```python
from build123d import *

# Parameters (mm, degrees)
SKETCH1_R             = 43
BOSS_EXTRUDE1_DEPTH   = 20
SKETCH2_R             = 44
BOSS_EXTRUDE2_DEPTH   = 8
FILLET1_R             = 20
BOSS_EXTRUDE3_DEPTH   = 10
SKETCH5_R             = 2.1
CUT_EXTRUDE1_DEPTH    = 4
CUT_EXTRUDE2_DEPTH    = 5
FILLET2_R             = 3
BOSS_EXTRUDE4_DEPTH   = 10
SKETCH10_R            = 2.1
CUT_EXTRUDE3_DEPTH    = 4
SKETCH11_R            = 3.25
CUT_EXTRUDE4_DEPTH    = 47
CROQUIS1_R            = 2.75
CORTAR_EXTRUIR1_DEPTH = 13
CROQUIS2_R            = 6.4
CORTAR_EXTRUIR2_DEPTH = 10


with BuildPart() as part:
    # Sketch1 → Boss-Extrude1 (new body)
    with BuildSketch(Plane(origin=(0, 0, 0), x_dir=(1, 0, 0), z_dir=(0, 1, 0))):
        with Locations(Location((0, 0, 0), (0, 0, 270))):
            Circle(SKETCH1_R)
    extrude(amount=BOSS_EXTRUDE1_DEPTH)

    # Sketch2 → Boss-Extrude2 (add)
    with BuildSketch(Plane(origin=(0, 20, 0), x_dir=(1, 0, 0), z_dir=(0, 1, 0))):
        with Locations(Location((0, 0, 0), (0, 0, 270))):
            Circle(SKETCH2_R)
    extrude(amount=-BOSS_EXTRUDE2_DEPTH)

    # Fillet1
    # the kernel refuses this fillet: 20 mm, written as the material it adds along each edge
    with BuildSketch(Plane(origin=(0, 12, 0), x_dir=(0, 0, 1), z_dir=(1, 0, 0))) as fillet1_piece_1:
        with BuildLine():
            CenterArc((63, 6.244997998), FILLET1_R, 180, 18.194872339)
            Line((44, 0), (43, 0))
            Line((43, 0), (43, 6.244997998))
        make_face()
    revolve(axis=Axis((0, 12, 0), (0, -1, 0)))

    # Sketch4 → Boss-Extrude3 (add)
    with BuildSketch(Plane.XZ):
        Polygon((28.890073358, 11), (35.011581558, 11), (0, -38.567688166), (-2.046413556, -32.798368085), align=None)
    extrude(amount=BOSS_EXTRUDE3_DEPTH)

    # Sketch5 → Cut-Extrude1 (cut)
    with BuildSketch(Plane(origin=(18.174388611, 0, -12.837275908), x_dir=(-0.576932008090494, 0, -0.8167921755505927), z_dir=(0.8167921755505927, 0, -0.576932008090494))):
        with Locations((-21.184015986, -5)):
            Circle(SKETCH5_R)
        with Locations(Location((23.501785923, -5, 0), (0, 0, 180))):
            Circle(SKETCH5_R)
    extrude(amount=-CUT_EXTRUDE1_DEPTH, mode=Mode.SUBTRACT)

    # Sketch7 → Cut-Extrude2 (cut)
    with BuildSketch(Plane.XZ):
        with BuildLine():
            Line((8.455950561, -5.839980603), (-5.151807084, 3.771706651))
            ThreePointArc((-5.151807084, 3.771706651), (-8.391785298, 4.503949914), (-11.200570041, 2.730713525))
            Line((-11.200570041, 2.730713525), (-20.812257296, -10.87704412))
            ThreePointArc((-20.812257296, -10.87704412), (-21.544500559, -14.117022334), (-19.771264169, -16.925807077))
            Line((-19.771264169, -16.925807077), (-6.163506524, -26.537494332))
            ThreePointArc((-6.163506524, -26.537494332), (-2.92352831, -27.269737595), (-0.114743567, -25.496501205))
            Line((-0.114743567, -25.496501205), (9.496943688, -11.88874356))
            ThreePointArc((9.496943688, -11.88874356), (10.22918695, -8.648765346), (8.455950561, -5.839980603))
        make_face()
    extrude(amount=-CUT_EXTRUDE2_DEPTH, mode=Mode.SUBTRACT)

    # Fillet2
    fillet2_edges = [part.edges().sort_by_distance(p)[0] for p in [
        (0, 20, -44),
    ]]
    fillet(fillet2_edges, radius=FILLET2_R)

    # Sketch8 → Boss-Extrude4 (add)
    with BuildSketch(Plane.XZ):
        Polygon((28.890073358, 11), (-35.011581558, 11), (-31.47988754, 6), (25.35837934, 6), align=None)
    extrude(amount=BOSS_EXTRUDE4_DEPTH)

    # Sketch10 → Cut-Extrude3 (cut)
    with BuildSketch(Plane.XY.offset(11)):
        with Locations((-17.011581558, -5)):
            Circle(SKETCH10_R)
        with Locations((17.011581558, -5)):
            Circle(SKETCH10_R)
    extrude(amount=-CUT_EXTRUDE3_DEPTH, mode=Mode.SUBTRACT)

    # Sketch11 → Cut-Extrude4 (cut)
    with BuildSketch(Plane.XZ):
        with Locations(Location((0, 25, 0), (0, 0, 270))):
            Circle(SKETCH11_R)
    extrude(amount=-CUT_EXTRUDE4_DEPTH, mode=Mode.SUBTRACT)

    # Croquis1 → Cortar-Extruir1 (cut)
    with BuildSketch(Plane(origin=(0, 20, 0), x_dir=(1, 0, 0), z_dir=(0, 1, 0))):
        with Locations(Location((-15, 25, 0), (0, 0, 270))):
            Circle(CROQUIS1_R)
        with Locations(Location((15, 25, 0), (0, 0, 270))):
            Circle(CROQUIS1_R)
        with Locations(Location((15, -25, 0), (0, 0, 270))):
            Circle(CROQUIS1_R)
        with Locations(Location((-15, -25, 0), (0, 0, 270))):
            Circle(CROQUIS1_R)
    extrude(amount=-CORTAR_EXTRUIR1_DEPTH, mode=Mode.SUBTRACT)

    # Croquis2 → Cortar-Extruir2 (cut)
    with BuildSketch(Plane(origin=(0, 20, 0), x_dir=(1, 0, 0), z_dir=(0, 1, 0))):
        with Locations(Location((0, 0, 0), (0, 0, 270))):
            Circle(CROQUIS2_R)
    extrude(amount=-CORTAR_EXTRUIR2_DEPTH, mode=Mode.SUBTRACT)


solid = part.part
```
Can you work these out from the model? Positions are in its coordinate system, mm. A direction names the side the tool comes from. Round coordinates to 2 decimals unless told otherwise and drop trailing zeros. Loops run counter-clockwise (first coordinate to the right, second up) from the corner with the lowest first, then second, coordinate; pieces in that order, holes last. Notation, with made-up numbers: (9, 50) -> (31, 50) arc R31 ccw to (31, 81) -> close; hole circle Ø6 at (48.25, 76). An arc over 180 degrees is marked (long way). One line per item, written item: value. Start each with the question number.
1. If I drill on probe 1 along X at (y, z) = (14.75, 0); probe 2 along Z at (x, y) = (-2.5, 13.25); probe 3 along X at (y, z) = (11.5, -25), over which ranges is the centre line in solid material (lowest first)?
2. If we section it at B-B, the plane z = 0: Write out the boundary of the cut face in (x, y) (3 decimals), then the cut area to 3 significant figures.
3. If we section it at A-A, the plane y = -5: Write out the boundary of the cut face in (x, z).
4. For pin 1 (6.5 mm diameter, centred on x = 17.01, y = -5, fed in from -Z); pin 2 (5 mm diameter, centred on y = -1.5, z = 10, fed in from +X); pin 3 (1.5 mm diameter, centred on x = -32, y = 8.5, fed in from -Z), each with a flat end and sliding along its axis, tell me the tip position at first contact or that it passes through.
5. For faces 5 (the cylindrical face through (-16.04, -6.86, 9.03)), 6 (the flat face through (11.464, -4.93, -13.671)), 7 (the flat face through (-6, 5, -11)), 8 (the flat face through (27.15, -4.97, 6.8)), 9 (the cylindrical face through (15.121, 13.591, 22.253)), which set-ups out of +Z, -Z, +X, -X, +Y, -Y let a thin tool reach every point of the face, with its end or its side?
6. If we mould it in two halves opening along X, with no side actions, what happens to faces 1 (the cylindrical face through (-3.89, 15.07, -5.08)), 2 (the cylindrical face through (-2.971, 2.465, -27.278)), 3 (the flat face through (8, -10, 7)), 4 (the flat face through (-33.27, -4.93, 8.535))? For each: pulls with the +X half, pulls with the -X half, needs draft (parallel to the pull), parting line crosses it, or undercut.
Calculated:
1. probe 1: x = -44 to -6.4, 6.4 to 44
1. probe 2: z = -43.93 to -5.89, 5.89 to 22.92, 27.08 to 43.93
1. probe 3: x = -36.02 to -17.75, -12.25 to 12.25, 17.75 to 36.02
2. outline: (-44, 12) arc R20 cw to (-43, 5.755) -> (-43, 0) -> (-13.129, 0) -> (-13.129, 5) -> (0.188, 5) -> (0.188, 0) -> (21.12, 0) -> (21.12, -10) -> (27.242, -10) -> (27.242, 0) -> (43, 0) -> (43, 5.755) arc R20 cw to (44, 12) -> (44, 17) arc R3 ccw to (41, 20) -> (6.4, 20) -> (6.4, 10) -> (-6.4, 10) -> (-6.4, 20) -> (-41, 20) arc R3 ccw to (-44, 17) -> close
2. area: 1,600 mm²
3. outline: (-35.01, 11) -> (-31.48, 6) -> (25.36, 6) -> (-2.05, -32.8) -> (0, -38.57) -> (3.4, -33.75) -> (0.14, -31.44) -> (2.56, -28.01) -> (5.83, -30.32) -> (29.18, 2.75) -> (25.92, 5.06) -> (28.34, 8.49) -> (31.61, 6.18) -> (35.01, 11) -> (19.11, 11) -> (19.11, 7) -> (14.91, 7) -> (14.91, 11) -> (-14.91, 11) -> (-14.91, 7) -> (-19.11, 7) -> (-19.11, 11) -> close
4. pin 1: stops at z = -19.09
4. pin 2: stops at x = 42.25
4. pin 3: stops at z = -29.83
5. face 5: +Z
5. face 6: -X, -Y
5. face 7: -Y
5. face 8: none
5. face 9: +Y
6. face 1: undercut
6. face 2: undercut
6. face 3: needs draft
6. face 4: pulls with the -X half
